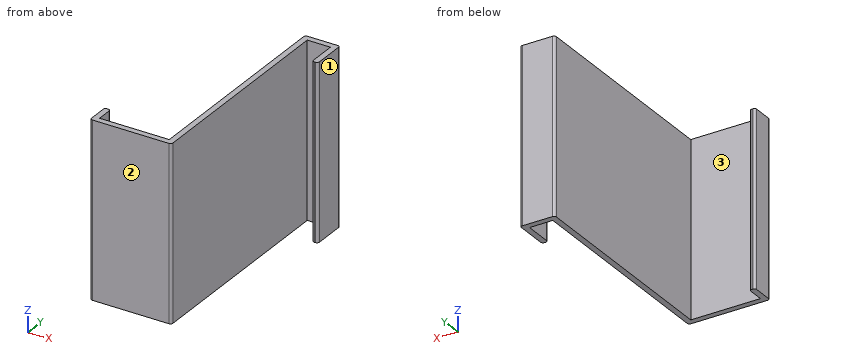
from build123d import *

# Parameters (mm, degrees)
F0_W     = 2.5
F0_H     = 6.25
F1_DEPTH = 75
F2_R     = 1
F3_R     = 1


with BuildPart() as f1:
    # F0 (on Top) → F1 (new body)
    with BuildSketch(Plane.XY):
        Polygon((2.5, 0), (0, 0), (0, -55.470833), (-15, -55.470833), (-15, -57.970833), (2.5, -57.970833), align=None)
        Polygon((7.5, 34.529167), (7.5, 37.029167), (0, 37.029167), (0, 0), (2.5, 0), (2.5, 34.529167), align=None)
        Polygon((12.5, 28.279167), (15, 28.279167), (15, 37.029167), (7.5, 37.029167), (7.5, 34.529167), (12.5, 34.529167), align=None)
        with Locations((13.75, 25.154167)):
            Rectangle(F0_W, F0_H)
        Polygon((-15, -57.970833), (-15, -55.470833), (-30, -55.470833), (-30, -47.970833), (-32.5, -47.970833), (-32.5, -57.970833), align=None)
    extrude(amount=F1_DEPTH)

    # F2
    f2_edges = [f1.edges().sort_by_distance(p)[0] for p in [
        (-32.5, -57.970833, 37.5),
        (2.5, -57.970833, 37.5),
        (15, 37.029167, 37.5),
        (0, 37.029167, 37.5),
    ]]
    fillet(f2_edges, radius=F2_R)

    # F3
    f3_edges = [f1.edges().sort_by_distance(p)[0] for p in [
        (-30, -47.970833, 37.5),
        (-32.5, -47.970833, 37.5),
        (15, 22.029167, 37.5),
        (12.5, 22.029167, 37.5),
    ]]
    fillet(f3_edges, radius=F3_R)


solid = f1.part
The model under review builds one solid part; all positions refer to its coordinate system, in mm. Face numbers are marked on the shaded views. Round coordinates to 2 decimals unless told otherwise and drop trailing zeros. Loops run counter-clockwise (first coordinate to the right, second up) from the corner with the lowest first, then second, coordinate; pieces in that order, holes last. Notation, with made-up numbers: (24.25, 67.5) -> (82.25, 67.5) arc R17 ccw to (82.25, 100.5) -> close; hole circle Ø2 at (-21.75, 48). An arc over 180 degrees is marked (long way). Return JSON: item names as keys, results as strings.
(1) For line 1 (X direction, y = 33.5, z = 18); line 2 (X direction, y = -20.5, z = 38); line 3 (Y direction, x = -31, z = 62), list the stretches that pass through material, from the lowest coordinate up.
Solved:
{"line 1": "0 to 2.5, 12.5 to 15", "line 2": "0 to 2.5", "line 3": "-57.97 to -47.97"}
(2) Add section C-C on x = -23.5. Write out the cut boundary in (y, z).
Solved:
{"outline": "(-57.97, 0) -> (-55.47, 0) -> (-55.47, 75) -> (-57.97, 75) -> close"}
(3) The part is to be moulded in two halves that separate along X. For the marked faces 1, 2 and 3, say which applies: released by +X, released by -X, zero draft, split by the parting line, or undercut.
Solved:
{"face 1": "released by +X", "face 2": "zero draft", "face 3": "undercut"}
(4) For pin 1 (10 mm diameter, centred on y = -40.5, z = 19, fed in from -X); pin 2 (12 mm diameter, centred on y = -44.5, z = 42, fed in from -X); pin 3 (22.5 mm diameter, centred on y = -29, z = 55, fed in from +X); pin 4 (5 mm diameter, centred on x = 7, z = 56, fed in from -Y), all flat-tipped, find the tip position at first contact; note any pin that passes through.
Solved:
{"pin 1": "x = 0", "pin 2": "x = -32.5", "pin 3": "x = 2.5", "pin 4": "y = 34.53"}
(5) Add section B-B on y = -43. Write out the cut boundary in (x, z).
Solved:
{"outline": "(0, 0) -> (2.5, 0) -> (2.5, 75) -> (0, 75) -> close"}
(6) Add section A-A on z = 62. Write out the cut boundary in (x, y).
Solved:
{"outline": "(-32.5, -56.97) arc R1 ccw to (-31.5, -57.97) -> (1.5, -57.97) arc R1 ccw to (2.5, -56.97) -> (2.5, 34.53) -> (12.5, 34.53) -> (12.5, 23.03) arc R1 ccw to (13.5, 22.03) -> (14, 22.03) arc R1 ccw to (15, 23.03) -> (15, 36.03) arc R1 ccw to (14, 37.03) -> (1, 37.03) arc R1 ccw to (0, 36.03) -> (0, -55.47) -> (-30, -55.47) -> (-30, -48.97) arc R1 ccw to (-31, -47.97) -> (-31.5, -47.97) arc R1 ccw to (-32.5, -48.97) -> close"}
